The drawing under review shows one solid part. Ordinate dimensions are in mm from its lowest x, y, z. Give positions to 0.01 mm unless a question says otherwise; leave off trailing zeros. Order: outer loops, then holes, each group sorted by start corner. A loop starts at its lowest first (then second) coordinate and runs counter-clockwise, first axis right, second up. Notation, with made-up numbers: (83, 38.5) -> (99, 38.5) arc R25 ccw to (99, 67.5) -> close; hole circle Ø7 at (-36.5, 83). An arc over 180 degrees is marked (long way). One line per item, written item: value. Start each with the question number.
1) Wall thickness on line 1 along X through (y, z) = (24.2, 69.85); line 2 along Y through (x, z) = (43.5, 65.5) (1 decimal); line 3 along X through (y, z) = (24.75, 57.15): over which ranges is each line inside the solid? List them lowest first. Write a range as from..to.
2) Consider section C-C (y = 14). State the section outline as (x, z) points (1 decimal), plus the area to 3 significant figures.
3) Consider section D-D (x = 25.4). State the section outline as (y, z) points (1 decimal).
4) For pin 1 (5.5 mm diameter, centred on y = 11, z = 24.5, fed in from +X) (3 decimals); pin 2 (4 mm diameter, centred on x = 43.5, y = 4.5, fed in from +Z); pin 3 (6 mm diameter, centred on x = 39.5, y = 22, fed in from -Z), all flat-tipped, find the tip position at first contact; note any pin that passes through.
5) Consider section B-B (z = 57.15). State the section outline as (x, y) points (1 decimal), plus the area to 3 significant figures.
6) Consider section A-A (x = 5). State the section outline as (y, z) points (1 decimal), plus the area to 3 significant figures.
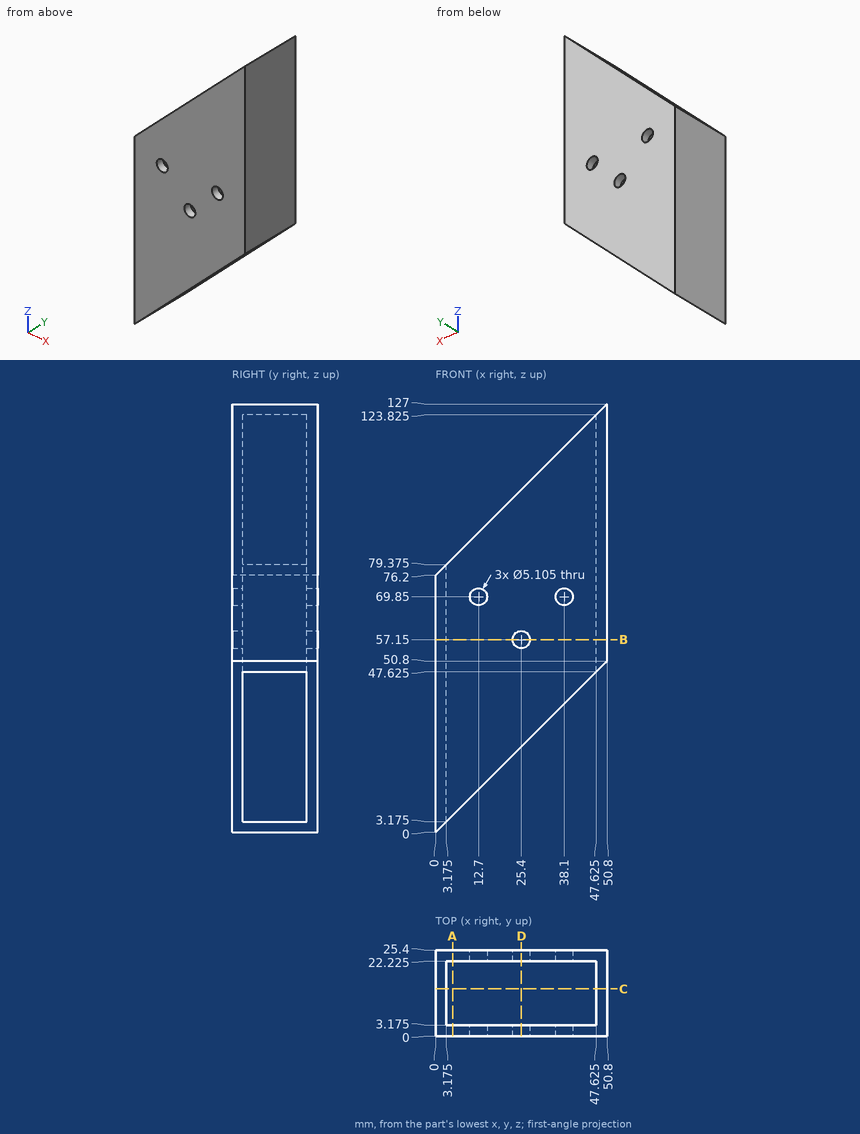
Checked values:
1. line 1: x = 0..10.15, 15.25..35.55, 40.65..50.8
1. line 2: y = 0..3.2, 22.2..25.4
1. line 3: x = 0..22.85, 27.95..50.8
2. outline: (0, 0) -> (3.2, 3.2) -> (3.2, 79.4) -> (0, 76.2) -> close; (47.6, 47.6) -> (50.8, 50.8) -> (50.8, 127) -> (47.6, 123.8) -> close
2. area: 484 mm^2
3. outline: (0, 25.4) -> (3.2, 25.4) -> (3.2, 54.6) -> (0, 54.6) -> close; (0, 59.7) -> (3.2, 59.7) -> (3.2, 101.6) -> (0, 101.6) -> close; (22.2, 25.4) -> (25.4, 25.4) -> (25.4, 54.6) -> (22.2, 54.6) -> close; (22.2, 59.7) -> (25.4, 59.7) -> (25.4, 101.6) -> (22.2, 101.6) -> close
4. pin 1: stops at x = 3.175
4. pin 2: stops at z = 121.2
4. pin 3: stops at z = 36.51
5. outline: (0, 0) -> (22.8, 0) -> (22.8, 3.2) -> (3.2, 3.2) -> (3.2, 22.2) -> (22.8, 22.2) -> (22.8, 25.4) -> (0, 25.4) -> close; (28, 0) -> (50.8, 0) -> (50.8, 25.4) -> (28, 25.4) -> (28, 22.2) -> (47.6, 22.2) -> (47.6, 3.2) -> (28, 3.2) -> close
5. area: 411 mm^2
6. outline: (0, 5) -> (3.2, 5) -> (3.2, 81.2) -> (0, 81.2) -> close; (22.2, 5) -> (25.4, 5) -> (25.4, 81.2) -> (22.2, 81.2) -> close
6. area: 484 mm^2
